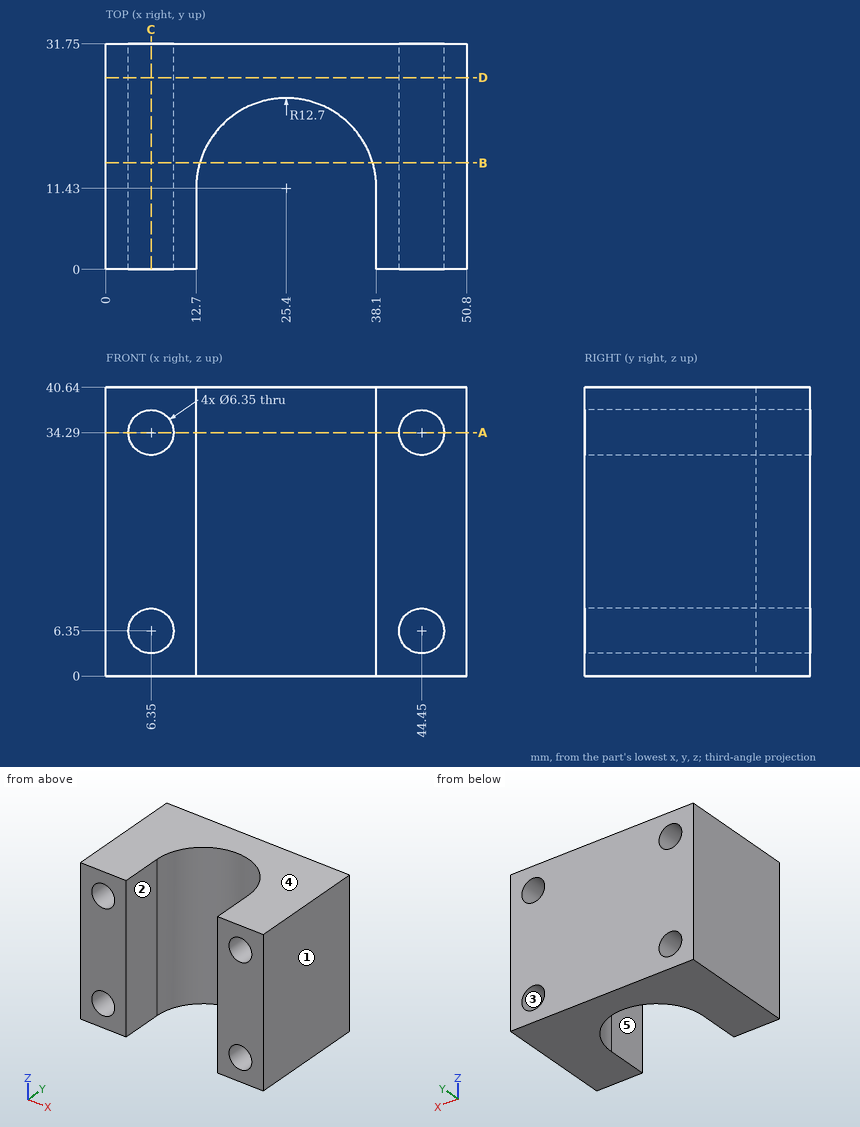
Answer from the drawing. Dimensions are ordinates in mm from the lowest x, y and z of the part. A direction names the side the tool comes from. Coordinates: 2 decimals unless noted, no trailing zeros. Loops run counter-clockwise (first coordinate to the right, second up) from the corner with the lowest first, then second, coordinate; pieces in that order, holes last. Notation, with made-up numbers: (36, 45.25) -> (51, 45.25) arc R37 cw to (51, 84.25) -> close; hole circle Ø2 at (83.5, 20). An arc over 180 degrees is marked (long way). Return JSON: item names as keys, results as strings.
Item 1: Find section B-B (y = 15). Determine the outline of the cut face in (x, z) (3 decimals).
Answers:
{"outline": "(0, 0) -> (13.212, 0) -> (13.212, 40.64) -> (0, 40.64) -> close; (37.588, 0) -> (50.8, 0) -> (50.8, 40.64) -> (37.588, 40.64) -> close; hole circle Ø6.35 at (6.35, 6.35); hole circle Ø6.35 at (6.35, 34.29); hole circle Ø6.35 at (44.45, 6.35); hole circle Ø6.35 at (44.45, 34.29)"}
Item 2: Find section A-A (z = 34.29). Determine the outline of the cut face in (x, y) (3 decimals).
Answers:
{"outline": "(0, 0) -> (3.175, 0) -> (3.175, 31.75) -> (0, 31.75) -> close; (9.525, 0) -> (12.7, 0) -> (12.7, 11.43) arc R12.7 cw to (38.1, 11.43) -> (38.1, 0) -> (41.275, 0) -> (41.275, 31.75) -> (9.525, 31.75) -> close; (47.625, 0) -> (50.8, 0) -> (50.8, 31.75) -> (47.625, 31.75) -> close"}
Item 3: Find section D-D (y = 27). Determine the outline of the cut face in (x, z) (3 decimals).
Answers:
{"outline": "(0, 0) -> (50.8, 0) -> (50.8, 40.64) -> (0, 40.64) -> close; hole circle Ø6.35 at (6.35, 6.35); hole circle Ø6.35 at (6.35, 34.29); hole circle Ø6.35 at (44.45, 6.35); hole circle Ø6.35 at (44.45, 34.29)"}
Item 4: Find the intervals of material crossed by probe 1 along X at (y, z) = (27, 6.5); probe 2 along X at (y, z) = (22, 34); probe 3 along X at (y, z) = (3, 8), in increasing order.
Answers:
{"probe 1": "x = 0 to 3.18, 9.52 to 41.28, 47.62 to 50.8", "probe 2": "x = 0 to 3.19, 9.51 to 18.36, 32.44 to 41.29, 47.61 to 50.8", "probe 3": "x = 0 to 3.64, 9.06 to 12.7, 38.1 to 41.74, 47.16 to 50.8"}
Item 5: A flat-ended cylindrical pin translates along its axis: P1, Ø1, axis at x = 27, z = 11, coming from the -Y side. Find the tip coordinate at first contact, or state that the pin passes through.
Answers:
{"P1": "stops at y = 23.96"}
Item 6: For the marked faces 1 and 2, determine the directions among +Z, -Z, +X, -X, +Y, -Y from which every point of the face is accessible in a straight line to the end or side of a thin tool.
Answers:
{"face 1": "+Z, -Z, +X, +Y, -Y", "face 2": "+Z, -Z, -Y"}
Item 7: For a pull along Z with two mould halves and no side action, classify the marked faces 3, 4 and 5 as +Z half, -Z half, draft (parallel to the pull), parting line (faces both ways), or undercut.
Answers:
{"face 3": "undercut", "face 4": "+Z half", "face 5": "draft"}
Item 8: Find section C-C (x = 6.35). Determine the outline of the cut face in (y, z) (3 decimals), plus the area to 3 significant figures.
Answers:
{"outline": "(0, 0) -> (31.75, 0) -> (31.75, 3.175) -> (0, 3.175) -> close; (0, 9.525) -> (31.75, 9.525) -> (31.75, 31.115) -> (0, 31.115) -> close; (0, 37.465) -> (31.75, 37.465) -> (31.75, 40.64) -> (0, 40.64) -> close", "area": "887 mm2"}
